```python
from build123d import *

# Parameters (mm, degrees)
SKETCH1_R           = 12.655
BOSS_EXTRUDE1_DEPTH = 20.2
BOSS_EXTRUDE2_DEPTH = 3.22
SKETCH3_R           = 2.875
CUT_EXTRUDE1_DEPTH  = 8.5


with BuildPart() as part:
    # Sketch1 → Boss-Extrude1 (new body)
    with BuildSketch(Plane(origin=(0, 0, 0), x_dir=(1, 0, 0), z_dir=(0, 1, 0))):
        with Locations(Location((0, 0, 0), (0, 0, 270))):
            Circle(SKETCH1_R)
    extrude(amount=BOSS_EXTRUDE1_DEPTH)

    # Sketch2 → Boss-Extrude2 (add)
    with BuildSketch(Plane(origin=(0, 20.2, 0), x_dir=(1, 0, 0), z_dir=(0, 1, 0))):
        with BuildLine():
            Line((1.600897841, 16.422153516), (0, 0))
            Line((0, 0), (-9.798866593, 13.275248151))
            ThreePointArc((-9.798866593, 13.275248151), (-4.390606594, 15.90511156), (1.600897841, 16.422153516))
        make_face()
    extrude(amount=-BOSS_EXTRUDE2_DEPTH)

    # Sketch3 → Cut-Extrude1 (cut)
    with BuildSketch(Plane(origin=(0, 20.2, 0), x_dir=(1, 0, 0), z_dir=(0, 1, 0))):
        with Locations(Location((0, 0, 0), (0, 0, 270))):
            Circle(SKETCH3_R)
    extrude(amount=-CUT_EXTRUDE1_DEPTH, mode=Mode.SUBTRACT)


solid = part.part
```
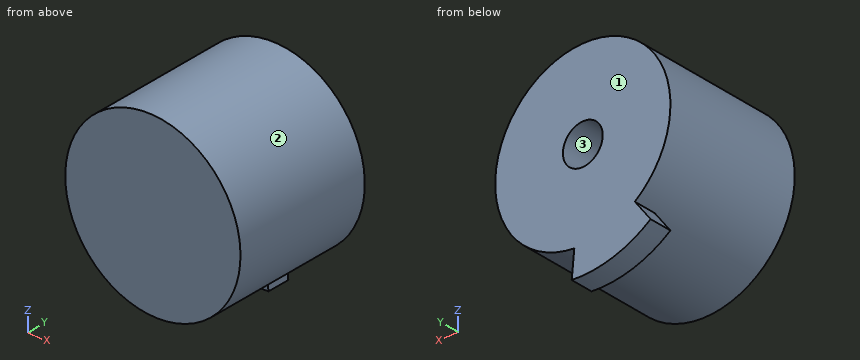
Input: part model. Units: mm. Frame: model coordinates. Face numbers are marked on the shaded views. Coordinates: 2 decimals unless noted, no trailing zeros. Loops run counter-clockwise (first coordinate to the right, second up) from the corner with the lowest first, then second, coordinate; pieces in that order, holes last. Notation, with made-up numbers: M 50.5,-30 L 104.5,-30 A28 ccw 104.5,-5 Z; hole C 81,57 d2. An arc over 180 degrees is marked long. One line per item, written item: value.
(1) Pull-direction query (X, two-part tool) for the marked faces 1, 2 and 3; classes: +X half, -X half, draft (parallel to the pull), parting line (faces both ways), or undercut.
Filled in:
face 1: draft
face 2: parting line
face 3: undercut
(2) Line query: line 1 along X through (y, z) = (18, 0) (3 decimals); line 2 along Z through (x, y) = (-2, 13.5); line 3 along X through (y, z) = (16.5, -1.75). Output: solid intervals per line, ascending. Write a range as from..to.
Filled in:
line 1: -12.655..-2.875, 2.875..12.655
line 2: -12.5..-2.07, 2.07..12.5
line 3: -12.53..-2.28, 2.28..12.53
(3) Section A-A (x = 0). Output: boundary loops of the cut face in (y, z) (3 decimals), and give its area (3 significant figures).
Filled in:
outline: M 0,-12.655 L 16.98,-12.655 L 16.98,-16.5 L 20.2,-16.5 L 20.2,-2.875 L 11.7,-2.875 L 11.7,2.875 L 20.2,2.875 L 20.2,12.655 L 0,12.655 Z
area: 475 mm^2
(4) Pin query (flat end, axial travel): pin 1 (3 mm diameter, centred on x = 4, y = 7, fed in from +Z); pin 2 (5 mm diameter, centred on x = 6, y = 7, fed in from +Z); pin 3 (3 mm diameter, centred on y = 13.5, z = 7.5, fed in from -X). Return the tip coordinate at first contact, or that it passes through.
Filled in:
pin 1: z = 12.41
pin 2: z = 12.16
pin 3: x = -11.14
(5) Section B-B (z = 0). Output: boundary loops of the cut face in (x, y) (3 decimals), and give its area (3 significant figures).
Filled in:
outline: M -12.655,0 L 12.655,0 L 12.655,20.2 L 2.875,20.2 L 2.875,11.7 L -2.875,11.7 L -2.875,20.2 L -12.655,20.2 Z
area: 462 mm^2
(6) Section D-D (y = 4.25). Output: boundary loops of the cut face in (x, z) (3 decimals).
Filled in:
outline: C 0,0 d25.31
(7) Section C-C (y = 15). Output: boundary loops of the cut face in (x, z) (3 decimals), and give its area (3 significant figures).
Filled in:
outline: C 0,0 d25.31; hole C 0,0 d5.75
area: 477 mm^2
